Input: dimensioned drawing with shaded views. Units: mm. Origin: part minimum x, y, z. A direction names the side the tool comes from. Coordinates: 2 decimals unless noted, no trailing zeros. Loops run counter-clockwise (first coordinate to the right, second up) from the corner with the lowest first, then second, coordinate; pieces in that order, holes last. Notation, with made-up numbers: (1.5, 36.5) - (25.5, 36.5) arc R20 cw to (25.5, 51.5) - close; hole circle Ø11 at (52, 1). An arc over 180 degrees is marked (long way). Write item = value, one per line. Start each with the question number.
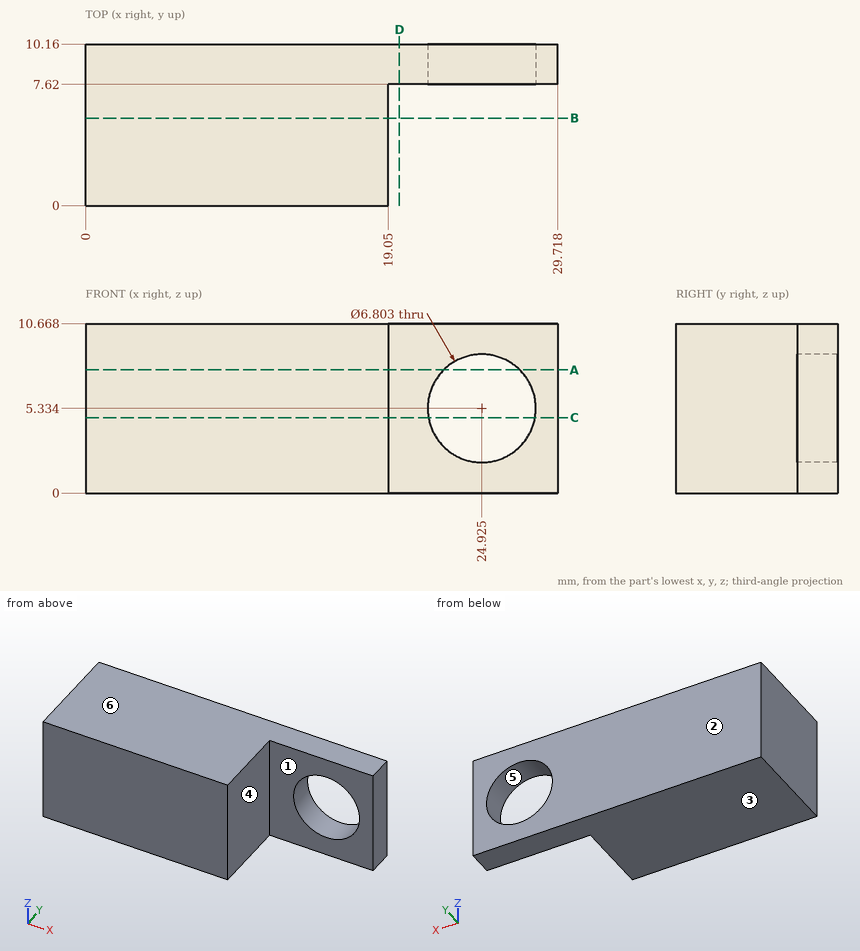
Item 1: Cut plane A-A on z = 7.75. Return loops of the section in (x, y).
Item 2: Cut plane B-B on y = 5.5. Return loops of the section in (x, z), plus the area to 3 significant figures.
Item 3: Access query for the marked faces 1 and 2. Directions: +Z, -Z, +X, -X, +Y, -Y. A direction counts if a zero-diameter tool reaches every point of the face in a straight line with its end or side. Return the directions, or none.
Item 4: Cut plane C-C on z = 4.75. Return loops of the section in (x, y), plus the area to 3 significant figures.
Item 5: Ray query, line 1 (X direction, y = 4.25, z = 3.5); line 2 (Y direction, x = 21.75, z = 9.75); line 3 (X direction, y = 9.75, z = 3). Return the intervals inside material, ascending.
Item 6: Cut plane D-D on x = 19.75. Return loops of the section in (y, z), plus the area to 3 significant figures.
Item 7: Pin query (flat end, axial travel): pin 1 (3 mm diameter, centred on x = 23, z = 6, fed in from -Y); pin 2 (2.5 mm diameter, centred on y = 3, z = 6.5, fed in from +X). Return the tip coordinate at first contact, or that it passes through.
Item 8: Pull-direction query (Z, two-part tool) for the marked faces 3, 4, 5 and 6; classes: pulls with the +Z half, pulls with the -Z half, needs draft (parallel to the pull), parting line crosses it, or undercut.
Recorded:
q1.outline = (0, 0) - (19.05, 0) - (19.05, 7.62) - (22.53, 7.62) - (22.53, 10.16) - (0, 10.16) - close; (27.32, 7.62) - (29.72, 7.62) - (29.72, 10.16) - (27.32, 10.16) - close
q2.outline = (0, 0) - (19.05, 0) - (19.05, 10.67) - (0, 10.67) - close
q2.area = 203 mm²
q3.face_1 = +Z, -Z, +X, -Y
q3.face_2 = +Z, -Z, +X, -X, +Y
q4.outline = (0, 0) - (19.05, 0) - (19.05, 7.62) - (21.57, 7.62) - (21.57, 10.16) - (0, 10.16) - close; (28.28, 7.62) - (29.72, 7.62) - (29.72, 10.16) - (28.28, 10.16) - close
q4.area = 204 mm²
q5.line_1 = 0 to 19.05
q5.line_2 = 7.62 to 10.16
q5.line_3 = 0 to 22.45, 27.4 to 29.72
q6.outline = (7.62, 0) - (10.16, 0) - (10.16, 10.67) - (7.62, 10.67) - close
q6.area = 27.1 mm²
q7.pin_1 = 7.62
q7.pin_2 = 19.05
q8.face_3 = pulls with the -Z half
q8.face_4 = needs draft
q8.face_5 = undercut
q8.face_6 = pulls with the +Z half
